Read the model definition and answer for the solid it produces. Units are mm, in the model's axes. A direction names the side the tool comes from. Give positions to 0.01 mm unless a question says otherwise; leave off trailing zeros. Loops run counter-clockwise (first coordinate to the right, second up) from the corner with the lowest first, then second, coordinate; pieces in that order, holes last. Notation, with made-up numbers: (33.25, 35) - (77.25, 35) arc R6 ccw to (77.25, 40) - close; hole circle Ø6 at (48.25, 83). An arc over 180 degrees is marked (long way). Write item = value, one per line.
```python
from build123d import *

# Parameters (mm, degrees)
SKETCH_1_R             = 40
SKETCH_1_R_2           = 30
SKETCH_1_R_3           = 2
SM_BASE_FLANGE_1_DEPTH = 0.7


# Read off the part's stored shape, not the designer's step: 边线-法兰2
# Sheet-metal steps are written as plain solids
with BuildPart() as part:
    # Sketch 1 → 基体-法兰1 (new body)
    with BuildSketch(Plane(origin=(0, 0, 0), x_dir=(1, 0, 0), z_dir=(0, 1, 0))):
        with Locations(Location((0, 0, 0), (0, 0, 270))):
            Circle(SKETCH_1_R)
        with Locations(Location((0, 0, 0), (0, 0, 270))):
            Circle(SKETCH_1_R_2, mode=Mode.SUBTRACT)
        with Locations(Location((-30.310889132, 17.5, 0), (0, 0, 270))):
            Circle(SKETCH_1_R_3, mode=Mode.SUBTRACT)
        with Locations(Location((0, -35, 0), (0, 0, 270))):
            Circle(SKETCH_1_R_3, mode=Mode.SUBTRACT)
        with Locations(Location((30.310889132, 17.5, 0), (0, 0, 270))):
            Circle(SKETCH_1_R_3, mode=Mode.SUBTRACT)
    extrude(amount=-SM_BASE_FLANGE_1_DEPTH)

    # 边线-法兰2 outline → 边线-法兰2 (revolve, cut)
    with BuildSketch(Plane.XY):
        with BuildLine():
            Line((30.022503561, 0), (30, 0))
            Line((30, 0), (30, -0.7))
            Line((30, -0.7), (30.9, -0.7))
            ThreePointArc((30.9, -0.7), (30.338751392, -0.503562364), (30.022503561, 0))
        make_face()
    revolve(axis=Axis((0, 0, 0), (0, 1, 0)), mode=Mode.SUBTRACT)

    # Sm Edge Flange 2 2 outline → Sm Edge Flange 2 2 (revolve)
    with BuildSketch(Plane.XY):
        with BuildLine():
            Line((30.7, 29.3), (30, 29.3))
            Line((30, 29.3), (30, 0.2))
            ThreePointArc((30, 0.2), (30.005643585, 0.099368978), (30.022503561, 0))
            Line((30.022503561, 0), (30.9, 0))
            ThreePointArc((30.9, 0), (30.758578644, 0.058578644), (30.7, 0.2))
            Line((30.7, 0.2), (30.7, 29.3))
        make_face()
    revolve(axis=Axis((0, 0, 0), (0, 1, 0)))


solid = part.part
```
1) A tool of negligible diameter and unlimited length cuts with its end or side. For faces 1 (the face through (-24, -0.7, 21)), 2 (the face through (-24, 0, 21)), from which of +Z, -Z, +X, -X, +Y, -Y can it reach the whole face along a straight path? Write none if from no direction.
Output:
face_1 = +Z, -Z, +X, -X, -Y
face_2 = +Y
2) A cutting plane is placed at B-B on y = 10.5. Determine the outline of the cut face in (x, z).
Output:
outline = circle Ø61.4 at (0, 0); hole circle Ø60 at (0, 0)
3) The mould has two halves that part along X. Classify faces 3 (the face through (6.7, 29.3, 29.4)), 4 (the face through (-39.05, -0.35, -8.67)), 5 (the face through (-28.328, -0.345, -17.76)): pulls with the +X half, pulls with the -X half, needs draft (parallel to the pull), parting line crosses it, or undercut.
Output:
face_3 = needs draft
face_4 = parting line crosses it
face_5 = undercut
4) A cutting plane is placed at D-D on z = -17.5. Give the number of separate pieces and of enclosed holes in the cut face, then the cut area to 3 significant figures.
Output:
separate_pieces = 4
enclosed_holes = 0
area = 60.4 mm²
5) Find the intervals of material crossed by probe 1 along X at (y, z) = (-0.15, -17.5); probe 2 along X at (y, z) = (6.75, -1); probe 3 along Z at (x, y) = (0, 15.5), in increasing order.
Output:
probe_1 = -35.97 to -32.31, -28.31 to -24.45, 24.45 to 28.31, 32.31 to 35.97
probe_2 = -30.68 to -29.98, 29.98 to 30.68
probe_3 = -30.7 to -30, 30 to 30.7
6) A cutting plane is placed at C-C on x = -34. Determine the outline of the cut face in (y, z), then the cut area to 3 significant figures.
Output:
outline = (-0.7, -21.07) - (0, -21.07) - (0, 21.07) - (-0.7, 21.07) - close
area = 29.5 mm²
7) A cutting plane is placed at A-A on z = 35. Determine the outline of the cut face in (x, y), then the cut area to 3 significant figures.
Output:
outline = (-19.36, -0.7) - (-2, -0.7) - (-2, 0) - (-19.36, 0) - close; (2, -0.7) - (19.36, -0.7) - (19.36, 0) - (2, 0) - close
area = 24.3 mm²
8) Each of these flat-tipped pins is pushed along its axis until it touches: P1, Ø12, axis at y = 26, z = 32, coming from the -X side; P2, Ø2, axis at y = 25, z = 13.5, coming from the -X side; P3, Ø8, axis at y = 9.5, z = -21, coming from the +X side. Where does it stop, or does it pass through?
Output:
P1 = -16.32
P2 = -28.04
P3 = 25.56
